```python
from build123d import *

# Parameters (mm, degrees)
F1_DEPTH  = 7
F3_DEPTH  = 1.75
F4_R      = 1.75
F5_DEPTH  = 5.25
F7_R      = 10
F8_R      = 5
F9_R      = 2
F10_R     = 2.875
F10_R_2   = 1.75
F11_DEPTH = 2.75
F12_R     = 1.75
F13_DEPTH = 2.75


with BuildPart() as f1:
    # F0 (on Front) → F1 (new body)
    with BuildSketch(Plane.XZ):
        Polygon((25, 0), (0, 0), (0, -37), (25, -39), align=None)
    extrude(amount=F1_DEPTH)

    # F2 (on face) → F3 (cut)
    with BuildSketch(Plane.XZ.offset(7)):
        Polygon((25, -34), (25, -5), (5, -5), (5, -32), align=None)
    extrude(amount=-F3_DEPTH, mode=Mode.SUBTRACT)

    # F4 (on face) → F5 (cut)
    with BuildSketch(Plane.XZ.offset(5.25)):
        with Locations((8, -19)):
            Circle(F4_R)
        with Locations((18, -19.5)):
            Circle(F4_R)
    extrude(amount=-F5_DEPTH, mode=Mode.SUBTRACT)

    # F6: F1 across face


with BuildPart() as f1_1:
    add(f1.part)
    add(f1.part.mirror(Plane(origin=(9.0064102564, -7, -19.0021367521), x_dir=(1, 0, 0), z_dir=(0, -1, 0))))

    # F7
    f7_edges = [f1_1.edges().sort_by_distance(p)[0] for p in [
        (0, -7, 0),
        (0, -7, -37),
    ]]
    fillet(f7_edges, radius=F7_R)

    # F8
    f8_edges = [f1_1.edges().sort_by_distance(p)[0] for p in [
        (17.5, -14, 0),
        (17.5, 0, 0),
    ]]
    fillet(f8_edges, radius=F8_R)

    # F9
    f9_edges = [f1_1.edges().sort_by_distance(p)[0] for p in [
        (25, -14, -19.492013),
    ]]
    fillet(f9_edges, radius=F9_R)

    # F10 (on face) → F11 (cut)
    with BuildSketch(Plane.XZ.offset(14)):
        with Locations((8, -19)):
            Circle(F10_R)
        with Locations((8, -19)):
            Circle(F10_R_2, mode=Mode.SUBTRACT)
        with Locations((18, -19.5)):
            Circle(F10_R)
        with Locations((18, -19.5)):
            Circle(F10_R_2, mode=Mode.SUBTRACT)
    extrude(amount=-F11_DEPTH, mode=Mode.SUBTRACT)

    # F12 (on face) → F13 (cut)
    with BuildSketch(Plane(origin=(0, 0, 0), x_dir=(-1, 0, 0), z_dir=(0, 1, 0))):
        Polygon((-16.4122867597, -16.75), (-19.5877132403, -16.75), (-21.1754264805, -19.5), (-19.5877132403, -22.25), (-16.4122867597, -22.25), (-14.8245735195, -19.5), align=None)
        with Locations((-18, -19.5)):
            Circle(F12_R, mode=Mode.SUBTRACT)
        Polygon((-6.4122867597, -16.25), (-9.5877132403, -16.25), (-11.1754264805, -19), (-9.5877132403, -21.75), (-6.4122867597, -21.75), (-5, -19.3038475773), (-5, -18.6961524227), align=None)
        with Locations((-8, -19)):
            Circle(F12_R, mode=Mode.SUBTRACT)
    extrude(amount=-F13_DEPTH, mode=Mode.SUBTRACT)


solid = f1_1.part
```
Build history of the part. All positions in model axes, mm. A direction names the side the tool comes from. Round coordinates to 2 decimals unless told otherwise and drop trailing zeros. Write each loop counter-clockwise with the first axis right and the second up, starting at its lowest first coordinate (ties: lowest second). Pieces come first, ordered by that corner, then holes. Notation, with made-up numbers: (6, 24.25) - (32, 24.25) arc R7 ccw to (32, 35.25) - close; hole circle Ø1 at (30.25, -20). An arc over 180 degrees is marked (long way). Write each question's results on one line, items separated by ' | '. Start each with the question number.
Item 1: Mould opens along Z. For faces 1 (the face through (20.39, -1.36, -20.86)), 2 (the face through (16.231, -1.504, -36.868)), 3 (the face through (5.696, -1.356, -17.49)), 4 (the face through (24.43, -13.4, -19.21)) say: pulls with the +Z half, pulls with the -Z half, needs draft (parallel to the pull), parting line crosses it, or undercut.
Item 2: Saw through at A-A (y = -5.75). Write the cut outline in (x, z).
Item 3: Wall check: L1, parallel to Y at x = 19, z = -30.5; L2, parallel to X at y = -8, z = -15.5; L3, parallel to Z at x = 18.25, y = -5. Give the ranges that are in metal, low to high. Write a range as [from, to].
Item 4: Drop flat-ended pins along their axis: P1, Ø6.5, axis at x = 8, z = -18.5, coming from the -Y side; P2, Ø4.5, axis at x = 18, z = -19.5, coming from the +Y side; P3, Ø3, axis at x = 17.5, y = -7.5, coming from the -Z side; P4, Ø0.8, axis at x = 18.5, y = -2, coming from the -Z side. Give the stop position or say it passes through.
Item 5: Which spindle directions (+Z, -Z, +X, -X, +Y, -Y) get a long thin tool onto all of the face, cutting with end or side? Do faces 5 (the face through (15, -8.75, -19)), 6 (the face through (18, -1, -16.75)), 7 (the face through (17.377, -12.644, -22.307)), 8 (the face through (3.01, -7.03, -2.85)). Say none if no direction does.
Results are:
1) face 1: undercut | face 2: pulls with the -Z half | face 3: undercut | face 4: needs draft
2) outline: (0, -27.77) arc R10 ccw to (9.2, -37.74) - (22.84, -38.83) arc R2 ccw to (25, -36.83) - (25, -34) - (5, -32) - (5, -5) - (25, -5) - (25, -2) arc R2 ccw to (23, 0) - (10, 0) arc R10 ccw to (0, -10) - close
3) L1: y = [-14, -8.75], [-5.25, 0] | L2: x = [0, 5] | L3: z = [-38.46, -21.23], [-17.77, 0]
4) P1: stops at y = -14 | P2: stops at y = -2.75 | P3: stops at z = -38.52 | P4: stops at z = -37.75
5) face 5: +X | face 6: +Y | face 7: -Y | face 8: +Z, -X, +Y, -Y
